from build123d import *

# Parameters (mm, degrees)
A_BASE_T42_OUTLINE_R        = 2.2479
A_BASE_T42_OUTLINE_R_2      = 1
A_BASE_T42_DEPTH            = 3
OUTER_BRIM_DEPTH            = 3
SKETCH5_W                   = 3
SKETCH5_H                   = 15
SKETCH5_W_2                 = 15
SKETCH5_H_2                 = 3
BASE_SUPPORTS_DEPTH         = 3
BASE_SUPPORTS_CHAMFER_SIZE  = 3
COVER_START                 = -3
SKETCH6_R                   = 1
COVER_DEPTH                 = 3
SKETCH7_W                   = 5
SKETCH7_H                   = 55.64
SERVO_SIDE_SUPPORTS_DEPTH   = 8.5
SKETCH8_W                   = 5
SKETCH8_H                   = 7.82
SERVO_SIDE_EXTENSIONS_DEPTH = 5
SERVO_CONTOURING_R          = 1


# Read off the part's stored shape, not the designer's step: a_base_t42
with BuildPart() as part:
    # a_base_t42 outline → a_base_t42 (new body)
    with BuildSketch(Plane(origin=(0, 0, 0), x_dir=(1, 0, 0), z_dir=(0, 1, 0))):
        with BuildLine():
            ThreePointArc((31.5, -42), (52.5, 0), (31.5, 42))
            Line((31.5, 42), (-31.5, 42))
            ThreePointArc((-31.5, 42), (-52.5, 0), (-31.5, -42))
            Line((-31.5, -42), (31.5, -42))
        make_face()
        with Locations((-23, -35)):
            Circle(A_BASE_T42_OUTLINE_R, mode=Mode.SUBTRACT)
        with Locations((23, -35)):
            Circle(A_BASE_T42_OUTLINE_R, mode=Mode.SUBTRACT)
        with Locations((-40.25, 0)):
            Circle(A_BASE_T42_OUTLINE_R_2, mode=Mode.SUBTRACT)
        with Locations((-23, 35)):
            Circle(A_BASE_T42_OUTLINE_R, mode=Mode.SUBTRACT)
        with Locations((40.25, 0)):
            Circle(A_BASE_T42_OUTLINE_R_2, mode=Mode.SUBTRACT)
        with Locations((23, 35)):
            Circle(A_BASE_T42_OUTLINE_R, mode=Mode.SUBTRACT)
    extrude(amount=A_BASE_T42_DEPTH)

    # Sketch1 → Outer Brim (add)
    with BuildSketch(Plane(origin=(0, 3, 0), x_dir=(1, 0, 0), z_dir=(0, 1, 0))):
        with BuildLine():
            Line((-31.5, -42), (31.5, -42))
            ThreePointArc((31.5, -42), (52.5, 0), (31.5, 42))
            Line((31.5, 42), (-31.5, 42))
            ThreePointArc((-31.5, 42), (-52.5, 0), (-31.5, -42))
        make_face()
        with BuildLine():
            Line((30.483602149, 39), (-30.483602149, 39))
            ThreePointArc((-30.483602149, 39), (-49.5, 0), (-30.483602149, -39))
            Line((-30.483602149, -39), (30.483602149, -39))
            ThreePointArc((30.483602149, -39), (49.5, 0), (30.483602149, 39))
        make_face(mode=Mode.SUBTRACT)
    extrude(amount=OUTER_BRIM_DEPTH)

    # Sketch5 → Base Supports (add)
    with BuildSketch(Plane(origin=(0, 3, 0), x_dir=(1, 0, 0), z_dir=(0, 1, 0))):
        with Locations((-34.325, -12.5)):
            Rectangle(SKETCH5_W, SKETCH5_H)
        with Locations((-34.325, 12.5)):
            Rectangle(SKETCH5_W, SKETCH5_H)
        with Locations((-25.325, -27)):
            Rectangle(SKETCH5_W_2, SKETCH5_H_2)
        with Locations((-25.325, 27)):
            Rectangle(SKETCH5_W_2, SKETCH5_H_2)
    extrude(amount=BASE_SUPPORTS_DEPTH)

    # Base Supports Chamfer
    base_supports_chamfer_edges = [part.edges().sort_by_distance(p)[0] for p in [
        (-25.325, 3, 28.5),
        (-25.325, 3, -28.5),
        (-35.825, 3, 12.5),
        (-35.825, 3, -12.5),
    ]]
    chamfer(base_supports_chamfer_edges, length=BASE_SUPPORTS_CHAMFER_SIZE - 0.0001)  # a hair under: the kernel refuses the full size

    # Sketch6 → Cover (add)
    with BuildSketch(Plane(origin=(0, 3, 0), x_dir=(1, 0, 0), z_dir=(0, 1, 0)).offset(COVER_START)):
        with Locations((-40.25, 0)):
            Circle(SKETCH6_R)
        with Locations((40.25, 0)):
            Circle(SKETCH6_R)
    extrude(amount=COVER_DEPTH)

    # Sketch7 → Servo Side Supports (add)
    with BuildSketch(Plane(origin=(0, 3, 0), x_dir=(1, 0, 0), z_dir=(0, 1, 0))):
        with Locations((2.425, 0)):
            Rectangle(SKETCH7_W, SKETCH7_H)
    extrude(amount=SERVO_SIDE_SUPPORTS_DEPTH)

    # Sketch8 → Servo Side Extensions (add)
    with BuildSketch(Plane(origin=(0, 11.5, 0), x_dir=(1, 0, 0), z_dir=(0, 1, 0))):
        with Locations((2.425, 23.91)):
            Rectangle(SKETCH8_W, SKETCH8_H)
        with Locations((2.425, -23.91)):
            Rectangle(SKETCH8_W, SKETCH8_H)
    extrude(amount=SERVO_SIDE_EXTENSIONS_DEPTH)

    # Servo Contouring
    servo_contouring_edges = [part.edges().sort_by_distance(p)[0] for p in [
        (2.425, 3, -27.82),
        (2.425, 16.5, -27.82),
        (2.425, 3, 27.82),
        (2.425, 16.5, 27.82),
        (2.425, 16.5, 20),
        (2.425, 16.5, -20),
    ]]
    fillet(servo_contouring_edges, radius=SERVO_CONTOURING_R)


solid = part.part
The listing builds one solid part. Answer for the finished solid, in the listing's coordinates (mm). A direction names the side the tool comes from. Coordinates: 2 decimals unless noted, no trailing zeros. Loops run counter-clockwise (first coordinate to the right, second up) from the corner with the lowest first, then second, coordinate; pieces in that order, holes last. Notation, with made-up numbers: M 79,-6.75 L 101,-6.75 A7 ccw 101,-0.75 Z; hole C -7,3.25 d7. An arc over 180 degrees is marked long. Answer in a Markdown table with one row per item.
1) Find section A-A (x = -23). Count the separate pieces of the cut face and the enclosed holes in it, then the cut area to 3 significant figures.
Answers below:
| item | result |
|---|---|
| separate pieces | 3 |
| enclosed holes | 0 |
| area | 270 mm^2 |
2) Given pin 1 (1.5 mm diameter, centred on x = 2, y = 11, fed in from +Z); pin 2 (5 mm diameter, centred on y = 13.5, z = -22, fed in from +X) (3 decimals); pin 3 (2.5 mm diameter, centred on x = -34.5, z = 14.5, fed in from +Y); pin 4 (2 mm diameter, centred on x = -35.5, z = 27, fed in from -Y), each flat-ended and moving along its own axis, determine where each tip first touches the part or whether it passes through.
Answers below:
| item | result |
|---|---|
| pin 1 | z = 27.82 |
| pin 2 | x = 4.925 |
| pin 3 | y = 6 |
| pin 4 | y = 0 |
3) Find section C-C (x = 2). Determine the outline of the cut face in (y, z).
Answers below:
| item | result |
|---|---|
| outline | M 0,-42 L 6,-42 L 6,-39 L 3,-39 L 3,-28.82 A1 cw 4,-27.82 L 15.5,-27.82 A1 ccw 16.5,-26.82 L 16.5,-21 A1 ccw 15.5,-20 L 11.5,-20 L 11.5,20 L 15.5,20 A1 ccw 16.5,21 L 16.5,26.82 A1 ccw 15.5,27.82 L 4,27.82 A1 cw 3,28.82 L 3,39 L 6,39 L 6,42 L 0,42 Z |
4) Find section B-B (y = 1.5). Determine the outline of the cut face in (x, z), then the cut area to 3 significant figures.
Answers below:
| item | result |
|---|---|
| outline | M -31.5,-42 L 31.5,-42 A52.5 ccw 31.5,42 L -31.5,42 A52.5 ccw Z; hole C -23,-35 d4.5; hole C -23,35 d4.5; hole C 23,-35 d4.5; hole C 23,35 d4.5 |
| area | 7,690 mm^2 |
5) Which of the six approach directions +Z, -Z, +X, -X, +Y, -Y give full straight-line access (tool end or side, diameter ignored) to faces 4 (the cylindrical face through (-23.29, 1.48, -37.23)), 5 (the flat face through (-25, 4, -25.5)), 6 (the flat face through (-34, 6, 12)), 7 (the flat face through (2, 13, -20))?
Answers below:
| item | result |
|---|---|
| face 4 | +Y, -Y |
| face 5 | +Y |
| face 6 | +Z, -Z, -X, +Y |
| face 7 | +X, -X, +Y |
6) Find the intervals of material crossed by probe 1 along Z at (x, y) = (23, 1.35); probe 2 along X at (y, z) = (3.25, 0.5) (3 decimals); probe 3 along X at (y, z) = (2.1, -35), in increasing order.
Answers below:
| item | result |
|---|---|
| probe 1 | -42 to -37.25, -32.75 to 32.75, 37.25 to 42 |
| probe 2 | -52.498 to -49.497, -0.075 to 4.925, 49.497 to 52.498 |
| probe 3 | -39.13 to -25.25, -20.75 to 20.75, 25.25 to 39.13 |
7) Determine the mould class of faces 1 (the flat face through (0, 3, 42)), 2 (the cylindrical face through (-24.657, 1.479, 33.481)), 3 (the flat face through (-34, 6, -13)) for opening direction Z: released by +Z, released by -Z, zero draft, split by the parting line, or undercut.
Answers below:
| item | result |
|---|---|
| face 1 | released by +Z |
| face 2 | undercut |
| face 3 | zero draft |
